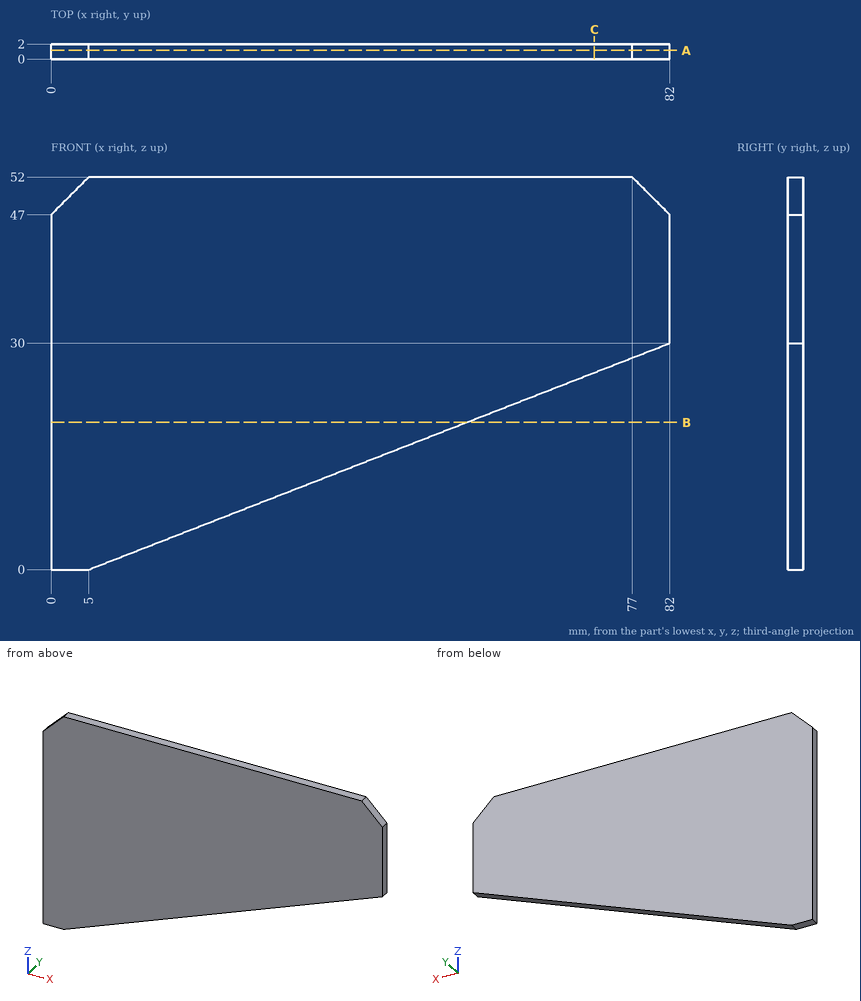
Print and shaded views of the part. All mm, measured from the part's lowest x, y and z. Coordinates: 2 decimals unless noted, no trailing zeros. Loops run counter-clockwise (first coordinate to the right, second up) from the corner with the lowest first, then second, coordinate; pieces in that order, holes last. Notation, with made-up numbers: (55, 43) - (108, 43) arc R27 ccw to (108, 59) - close; hole circle Ø5 at (71.5, 57). An arc over 180 degrees is marked (long way). Use one line per item in the form item = value. Start each with the question number.
1) Drill centre lines: L1, parallel to Z at x = 77.5, y = 1.05; L2, parallel to Z at x = 37, y = 0.1. Where is each one in solid material? Low to high. Write a range as from..to.
2) Band-saw the part on A-A (y = 1.15). Give the cut face in (x, z), and give its area (3 significant figures).
3) Flat gauge pin, fed straight in: pin 1 (5 mm diameter, centred on x = 13, z = 31.5, fed in from -Y). Where does the tip first touch, or does it go through?
4) Band-saw the part on B-B (z = 19.5). Give the cut face in (x, y).
5) Band-saw the part on C-C (x = 72). Give the cut face in (y, z), and give its area (3 significant figures).
Check values:
q1.L1 = 28.25..51.5
q1.L2 = 12.47..52
q2.outline = (0, 0) - (5, 0) - (82, 30) - (82, 47) - (77, 52) - (5, 52) - (0, 47) - close
q2.area = 3,080 mm2
q3.pin_1 = 0
q4.outline = (0, 0) - (55.05, 0) - (55.05, 2) - (0, 2) - close
q5.outline = (0, 26.1) - (2, 26.1) - (2, 52) - (0, 52) - close
q5.area = 51.8 mm2
